Source: CAD feature listing. Evaluate the final solid. Frame: model axes, mm. Coordinates: 2 decimals unless noted, no trailing zeros. Loops run counter-clockwise (first coordinate to the right, second up) from the corner with the lowest first, then second, coordinate; pieces in that order, holes last.
from build123d import *

# Parameters (mm, degrees)
BOSS_EXTRUDE1_DEPTH = 762
CUT_EXTRUDE1_DEPTH  = 763.26589161


with BuildPart() as part:
    # Sketch1 → Boss-Extrude1 (new body)
    with BuildSketch(Plane(origin=(0, 0, 0), x_dir=(0, 0, -1), z_dir=(1, 0, 0))):
        Polygon((0, 12.954), (0, -12.954), (-8.89, -12.954), (-8.89, -17.526), (-7.874, -17.526), (-7.874, -13.97), (0, -13.97), (0, -15.494), (1.016, -15.494), (1.016, 15.494), (0, 15.494), (0, 13.97), (-7.874, 13.97), (-7.874, 17.526), (-8.89, 17.526), (-8.89, 12.954), align=None)
    extrude(amount=BOSS_EXTRUDE1_DEPTH)

    # Sketch2 → Cut-Extrude1 (cut, through all)
    with BuildSketch(Plane(origin=(0, 0, -1.016), x_dir=(-1, 0, 0), z_dir=(0, 0, -1))):
        with BuildLine():
            Line((-749.554, 4.826), (-734.314, 4.826))
            ThreePointArc((-734.314, 4.826), (-729.488, 0), (-734.314, -4.826))
            Line((-734.314, -4.826), (-749.554, -4.826))
            ThreePointArc((-749.554, -4.826), (-754.38, 0), (-749.554, 4.826))
        make_face()
        with BuildLine():
            Line((-718.411391304, 4.826), (-703.171391304, 4.826))
            ThreePointArc((-703.171391304, 4.826), (-698.345391304, 0), (-703.171391304, -4.826))
            Line((-703.171391304, -4.826), (-718.411391304, -4.826))
            ThreePointArc((-718.411391304, -4.826), (-723.237391304, 0), (-718.411391304, 4.826))
        make_face()
        with BuildLine():
            Line((-687.268782609, 4.826), (-672.028782609, 4.826))
            ThreePointArc((-672.028782609, 4.826), (-667.202782609, 0), (-672.028782609, -4.826))
            Line((-672.028782609, -4.826), (-687.268782609, -4.826))
            ThreePointArc((-687.268782609, -4.826), (-692.094782609, 0), (-687.268782609, 4.826))
        make_face()
        with BuildLine():
            Line((-656.126173913, 4.826), (-640.886173913, 4.826))
            ThreePointArc((-640.886173913, 4.826), (-636.060173913, 0), (-640.886173913, -4.826))
            Line((-640.886173913, -4.826), (-656.126173913, -4.826))
            ThreePointArc((-656.126173913, -4.826), (-660.952173913, 0), (-656.126173913, 4.826))
        make_face()
        with BuildLine():
            Line((-624.983565217, 4.826), (-609.743565217, 4.826))
            ThreePointArc((-609.743565217, 4.826), (-604.917565217, 0), (-609.743565217, -4.826))
            Line((-609.743565217, -4.826), (-624.983565217, -4.826))
            ThreePointArc((-624.983565217, -4.826), (-629.809565217, 0), (-624.983565217, 4.826))
        make_face()
        with BuildLine():
            Line((-593.840956522, 4.826), (-578.600956522, 4.826))
            ThreePointArc((-578.600956522, 4.826), (-573.774956522, 0), (-578.600956522, -4.826))
            Line((-578.600956522, -4.826), (-593.840956522, -4.826))
            ThreePointArc((-593.840956522, -4.826), (-598.666956522, 0), (-593.840956522, 4.826))
        make_face()
        with BuildLine():
            Line((-562.698347826, 4.826), (-547.458347826, 4.826))
            ThreePointArc((-547.458347826, 4.826), (-542.632347826, 0), (-547.458347826, -4.826))
            Line((-547.458347826, -4.826), (-562.698347826, -4.826))
            ThreePointArc((-562.698347826, -4.826), (-567.524347826, 0), (-562.698347826, 4.826))
        make_face()
        with BuildLine():
            Line((-531.55573913, 4.826), (-516.31573913, 4.826))
            ThreePointArc((-516.31573913, 4.826), (-511.48973913, 0), (-516.31573913, -4.826))
            Line((-516.31573913, -4.826), (-531.55573913, -4.826))
            ThreePointArc((-531.55573913, -4.826), (-536.38173913, 0), (-531.55573913, 4.826))
        make_face()
        with BuildLine():
            Line((-500.413130435, 4.826), (-485.173130435, 4.826))
            ThreePointArc((-485.173130435, 4.826), (-480.347130435, 0), (-485.173130435, -4.826))
            Line((-485.173130435, -4.826), (-500.413130435, -4.826))
            ThreePointArc((-500.413130435, -4.826), (-505.239130435, 0), (-500.413130435, 4.826))
        make_face()
        with BuildLine():
            Line((-469.270521739, 4.826), (-454.030521739, 4.826))
            ThreePointArc((-454.030521739, 4.826), (-449.204521739, 0), (-454.030521739, -4.826))
            Line((-454.030521739, -4.826), (-469.270521739, -4.826))
            ThreePointArc((-469.270521739, -4.826), (-474.096521739, 0), (-469.270521739, 4.826))
        make_face()
        with BuildLine():
            Line((-438.127913043, 4.826), (-422.887913043, 4.826))
            ThreePointArc((-422.887913043, 4.826), (-418.061913043, 0), (-422.887913043, -4.826))
            Line((-422.887913043, -4.826), (-438.127913043, -4.826))
            ThreePointArc((-438.127913043, -4.826), (-442.953913043, 0), (-438.127913043, 4.826))
        make_face()
        with BuildLine():
            Line((-406.985304348, 4.826), (-391.745304348, 4.826))
            ThreePointArc((-391.745304348, 4.826), (-386.919304348, 0), (-391.745304348, -4.826))
            Line((-391.745304348, -4.826), (-406.985304348, -4.826))
            ThreePointArc((-406.985304348, -4.826), (-411.811304348, 0), (-406.985304348, 4.826))
        make_face()
        with BuildLine():
            Line((-375.842695652, 4.826), (-360.602695652, 4.826))
            ThreePointArc((-360.602695652, 4.826), (-355.776695652, 0), (-360.602695652, -4.826))
            Line((-360.602695652, -4.826), (-375.842695652, -4.826))
            ThreePointArc((-375.842695652, -4.826), (-380.668695652, 0), (-375.842695652, 4.826))
        make_face()
        with BuildLine():
            Line((-344.700086957, 4.826), (-329.460086957, 4.826))
            ThreePointArc((-329.460086957, 4.826), (-324.634086957, 0), (-329.460086957, -4.826))
            Line((-329.460086957, -4.826), (-344.700086957, -4.826))
            ThreePointArc((-344.700086957, -4.826), (-349.526086957, 0), (-344.700086957, 4.826))
        make_face()
        with BuildLine():
            Line((-313.557478261, 4.826), (-298.317478261, 4.826))
            ThreePointArc((-298.317478261, 4.826), (-293.491478261, 0), (-298.317478261, -4.826))
            Line((-298.317478261, -4.826), (-313.557478261, -4.826))
            ThreePointArc((-313.557478261, -4.826), (-318.383478261, 0), (-313.557478261, 4.826))
        make_face()
        with BuildLine():
            Line((-282.414869565, 4.826), (-267.174869565, 4.826))
            ThreePointArc((-267.174869565, 4.826), (-262.348869565, 0), (-267.174869565, -4.826))
            Line((-267.174869565, -4.826), (-282.414869565, -4.826))
            ThreePointArc((-282.414869565, -4.826), (-287.240869565, 0), (-282.414869565, 4.826))
        make_face()
        with BuildLine():
            Line((-251.27226087, 4.826), (-236.03226087, 4.826))
            ThreePointArc((-236.03226087, 4.826), (-231.20626087, 0), (-236.03226087, -4.826))
            Line((-236.03226087, -4.826), (-251.27226087, -4.826))
            ThreePointArc((-251.27226087, -4.826), (-256.09826087, 0), (-251.27226087, 4.826))
        make_face()
        with BuildLine():
            Line((-220.129652174, 4.826), (-204.889652174, 4.826))
            ThreePointArc((-204.889652174, 4.826), (-200.063652174, 0), (-204.889652174, -4.826))
            Line((-204.889652174, -4.826), (-220.129652174, -4.826))
            ThreePointArc((-220.129652174, -4.826), (-224.955652174, 0), (-220.129652174, 4.826))
        make_face()
        with BuildLine():
            Line((-188.987043478, 4.826), (-173.747043478, 4.826))
            ThreePointArc((-173.747043478, 4.826), (-168.921043478, 0), (-173.747043478, -4.826))
            Line((-173.747043478, -4.826), (-188.987043478, -4.826))
            ThreePointArc((-188.987043478, -4.826), (-193.813043478, 0), (-188.987043478, 4.826))
        make_face()
        with BuildLine():
            Line((-157.844434783, 4.826), (-142.604434783, 4.826))
            ThreePointArc((-142.604434783, 4.826), (-137.778434783, 0), (-142.604434783, -4.826))
            Line((-142.604434783, -4.826), (-157.844434783, -4.826))
            ThreePointArc((-157.844434783, -4.826), (-162.670434783, 0), (-157.844434783, 4.826))
        make_face()
        with BuildLine():
            Line((-126.701826087, 4.826), (-111.461826087, 4.826))
            ThreePointArc((-111.461826087, 4.826), (-106.635826087, 0), (-111.461826087, -4.826))
            Line((-111.461826087, -4.826), (-126.701826087, -4.826))
            ThreePointArc((-126.701826087, -4.826), (-131.527826087, 0), (-126.701826087, 4.826))
        make_face()
        with BuildLine():
            Line((-95.559217391, 4.826), (-80.319217391, 4.826))
            ThreePointArc((-80.319217391, 4.826), (-75.493217391, 0), (-80.319217391, -4.826))
            Line((-80.319217391, -4.826), (-95.559217391, -4.826))
            ThreePointArc((-95.559217391, -4.826), (-100.385217391, 0), (-95.559217391, 4.826))
        make_face()
        with BuildLine():
            Line((-64.416608696, 4.826), (-49.176608696, 4.826))
            ThreePointArc((-49.176608696, 4.826), (-44.350608696, 0), (-49.176608696, -4.826))
            Line((-49.176608696, -4.826), (-64.416608696, -4.826))
            ThreePointArc((-64.416608696, -4.826), (-69.242608696, 0), (-64.416608696, 4.826))
        make_face()
        with BuildLine():
            Line((-33.274, 4.826), (-18.034, 4.826))
            ThreePointArc((-18.034, 4.826), (-13.208, 0), (-18.034, -4.826))
            Line((-18.034, -4.826), (-33.274, -4.826))
            ThreePointArc((-33.274, -4.826), (-38.1, 0), (-33.274, 4.826))
        make_face()
    extrude(amount=-CUT_EXTRUDE1_DEPTH, mode=Mode.SUBTRACT)


solid = part.part
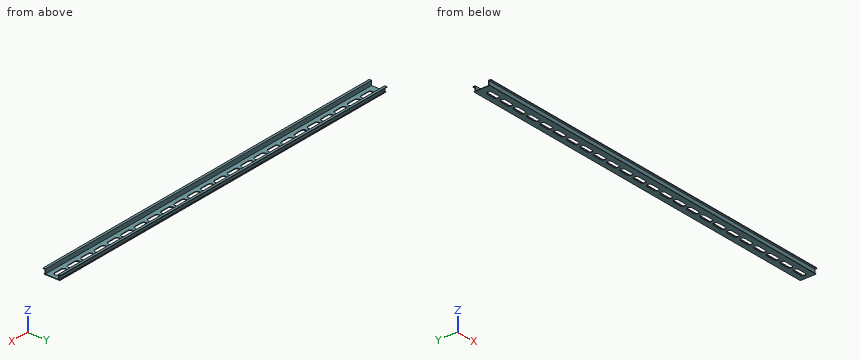
Q1. Section A-A, the plane z = 2.25. Return the cut outline in (x, y), plus the area to 3 significant figures.
Q2. Line query: line 1 along Y through (x, z) = (215, -0.5); line 2 along Y through (x, z) = (644.5, 2.25); line 3 along Z through (x, y) = (216.5, 7). Output: solid intervals per line, ascending.
Q3. Contact query for flat-ended pins moving along their axis: pin 1 Ø5 at (x, z) = (145, 5.5) entering from -Y; pin 2 Ø0.8 at (x, z) = (432, -0.5) entering from +Y; pin 3 Ø0.5 at (x, z) = (400.5, -0.5) entering from -Y; pin 4 Ø1 at (x, z) = (498, 4.5) entering from -Y. Output: stop coordinate, or through.
Derived:
1. outline: (0, -13.97) - (762, -13.97) - (762, -12.95) - (0, -12.95) - close; (0, 12.95) - (762, 12.95) - (762, 13.97) - (0, 13.97) - close
1. area: 1,550 mm2
2. line 1: y = -15.49 to -4.83, 4.83 to 15.49
2. line 2: y = -13.97 to -12.95, 12.95 to 13.97
2. line 3: z = -1.02 to 0
3. pin 1: stops at y = -17.53
3. pin 2: stops at y = 15.49
3. pin 3: stops at y = -15.49
3. pin 4: stops at y = -13.97
